```python
from build123d import *

# Parameters (mm, degrees)
EXTRUDE_1_DEPTH     = 20
FILLET_1_R          = 20
SKETCH_2_R          = 10
CUT_EXTRUDE_1_DEPTH = 68.586980995
EXTRUDE_2_DEPTH     = 8


with BuildPart() as part:
    # 草圖1 → 填料-伸長1 (new, symmetric)
    with BuildSketch(Plane.XY):
        Polygon((0, 0), (0, 30), (10, 30), (10, 12), (62, 12), (62, 0), align=None)
    extrude(amount=EXTRUDE_1_DEPTH, both=True)

    # 圓角1
    fillet_1_edges = [part.edges().sort_by_distance(p)[0] for p in [
        (62, 6, -20),
        (62, 6, 20),
    ]]
    fillet(fillet_1_edges, radius=FILLET_1_R - 0.0001)  # a hair under: the kernel refuses the full size

    # 草圖2 → 除料-伸長1 (cut, through all)
    with BuildSketch(Plane(origin=(0, 12, 0), x_dir=(1, 0, 0), z_dir=(0, 1, 0))):
        with Locations(Location((41.524228064, 0, 0), (0, 0, 270))):
            Circle(SKETCH_2_R)
    extrude(amount=-CUT_EXTRUDE_1_DEPTH, mode=Mode.SUBTRACT)

    # 草圖4 → 填料-伸長2 (add)
    with BuildSketch(Plane(origin=(0, 0, -20), x_dir=(-1, 0, 0), z_dir=(0, 0, -1))):
        Polygon((-10, 30), (-36, 12), (-10, 12), align=None)
    extrude(amount=-EXTRUDE_2_DEPTH)


solid = part.part
```
The model under review builds one solid part; all positions refer to its coordinate system, in mm. A direction names the side the tool comes from. Give positions to 0.01 mm unless a question says otherwise; leave off trailing zeros. Loops run counter-clockwise (first coordinate to the right, second up) from the corner with the lowest first, then second, coordinate; pieces in that order, holes last. Notation, with made-up numbers: (49, 88.5) - (60, 88.5) arc R17 cw to (60, 99.5) - close; hole circle Ø10 at (5, 75.5). An arc over 180 degrees is marked (long way). Answer as a JSON object with one key per item and string values.
Q1. Add section B-B on z = 9. State the section outline as (x, y) points.
Worked out:
{"outline": "(0, 0) - (37.17, 0) - (37.17, 12) - (10, 12) - (10, 30) - (0, 30) - close; (45.88, 0) - (59.86, 0) - (59.86, 12) - (45.88, 12) - close"}
Q2. To check wall thickness, follow line 1 along X through (y, z) = (3.25, 0); line 2 along Y through (x, z) = (38.5, 10); line 3 along Z through (x, y) = (13, 13.25). State the ranges of each line that lie inside material, in increasing order.
Worked out:
{"line 1": "x = 0 to 31.52, 51.52 to 62", "line 2": "y = 0 to 12", "line 3": "z = -20 to -12"}
Q3. Add section D-D on y = 25.5. State the section outline as (x, z) points, plus the area to 3 significant figures.
Worked out:
{"outline": "(0, -20) - (16.5, -20) - (16.5, -12) - (10, -12) - (10, 20) - (0, 20) - close", "area": "452 mm^2"}
Q4. Insertion check: pin 1 (6 mm diameter, centred on x = 41, z = 8.5, fed in from +Y); pin 2 (2 mm diameter, centred on y = 16.5, z = -7, fed in from +X). Each pin has a flat end and moves straight along its axis. Give the tip position at first contact, or say it passes through.
Worked out:
{"pin 1": "stops at y = 12", "pin 2": "stops at x = 10"}
Q5. Add section A-A on x = 47. State the section outline as (y, z) points.
Worked out:
{"outline": "(0, -19.36) - (12, -19.36) - (12, -8.37) - (0, -8.37) - close; (0, 8.37) - (12, 8.37) - (12, 19.36) - (0, 19.36) - close"}
Q6. For faces 1 (the flat face through (17, 12, -20)), 2 (the flat face through (30, 12, 5)), list the 3-axis set-ups (+Z, -Z, +X, -X, +Y, -Y) from which the entire face can be reached by the end or side of a thin tool; tool diameter is ignored.
Worked out:
{"face 1": "-Z, +X, -X, +Y, -Y", "face 2": "+Z, +X, +Y"}
Q7. Mouldability with a two-part tool opening along Z and no side actions: class faces 3 (the cylindrical face through (31.762, 6.084, -2.168)), 4 (the cylindrical face through (56.297, 5.916, -13.986)), 5 (the flat face through (25, 0, 0)) as +Z half, -Z half, draft (parallel to the pull), parting line (faces both ways), or undercut.
Worked out:
{"face 3": "undercut", "face 4": "-Z half", "face 5": "draft"}
